from build123d import *

# Parameters (mm, degrees)
SKETCH_W     = 105
SKETCH_H     = 70
PAD_DEPTH    = 5
SKETCH001_R  = 6.375
POCKET_DEPTH = 5
SKETCH002_R  = 1.2
HOLE_DEPTH   = 25


with BuildPart() as part:
    # Sketch → Pad (new body)
    with BuildSketch(Plane.XY):
        Rectangle(SKETCH_W, SKETCH_H)
    extrude(amount=PAD_DEPTH)

    # Sketch001 (on Face6 of Pad) → Pocket (cut)
    with BuildSketch(Plane.XY.offset(5)):
        with Locations((-33, 11)):
            Circle(SKETCH001_R)
        with Locations((33, 11)):
            Circle(SKETCH001_R)
        with Locations((33, -11)):
            Circle(SKETCH001_R)
        with Locations((-33, -11)):
            Circle(SKETCH001_R)
        with Locations((-11, 11)):
            Circle(SKETCH001_R)
        with Locations((11, 11)):
            Circle(SKETCH001_R)
        with Locations((-11, -11)):
            Circle(SKETCH001_R)
        with Locations((11, -11)):
            Circle(SKETCH001_R)
    extrude(amount=-POCKET_DEPTH, mode=Mode.SUBTRACT)

    # Sketch002 (on Face5 of Pocket) → Hole (cut)
    with BuildSketch(Plane.XY.offset(5)):
        with Locations((-47.5, 32.5)):
            Circle(SKETCH002_R)
        with Locations((47.5, 32.5)):
            Circle(SKETCH002_R)
        with Locations((-47.5, -32.5)):
            Circle(SKETCH002_R)
        with Locations((47.5, -32.5)):
            Circle(SKETCH002_R)
    extrude(amount=-HOLE_DEPTH, mode=Mode.SUBTRACT)


solid = part.part
Here's how the part is built. I have some questions about the finished solid (model axes, mm). Round coordinates to 2 decimals unless told otherwise and drop trailing zeros. Order: outer loops, then holes, each group sorted by start corner. A loop starts at its lowest first (then second) coordinate and runs counter-clockwise, first axis right, second up. Notation, with made-up numbers: (-15.75, 81) -> (-7.75, 81) arc R23 ccw to (-7.75, 96) -> close; hole circle Ø10 at (50.5, 73). An arc over 180 degrees is marked (long way). Return JSON: item names as keys, results as strings.
Q1. For pin 1 Ø11.5 at (x, y) = (11, 11) entering from +Z, with a flat end and sliding along its axis, tell me the tip position at first contact or that it passes through.
Filled sheet:
{"pin 1": "passes through"}
Q2. If we section it at B-B on z = 2.5: Give the number of separate pieces and of enclosed holes in the cut face, plus the area to 3 significant figures.
Filled sheet:
{"separate pieces": "1", "enclosed holes": "12", "area": "6,310 mm^2"}
Q3. If we section it at C-C on x = -47.5: List the corners of the cut face in (y, z) for me.
Filled sheet:
{"outline": "(-35, 0) -> (-33.7, 0) -> (-33.7, 5) -> (-35, 5) -> close; (-31.3, 0) -> (31.3, 0) -> (31.3, 5) -> (-31.3, 5) -> close; (33.7, 0) -> (35, 0) -> (35, 5) -> (33.7, 5) -> close"}
Q4. If we section it at D-D on y = 11: List the corners of the cut face in (x, z) for me (3 decimals), plus the area to 3 significant figures.
Filled sheet:
{"outline": "(-52.5, 0) -> (-39.375, 0) -> (-39.375, 5) -> (-52.5, 5) -> close; (-26.625, 0) -> (-17.375, 0) -> (-17.375, 5) -> (-26.625, 5) -> close; (-4.625, 0) -> (4.625, 0) -> (4.625, 5) -> (-4.625, 5) -> close; (17.375, 0) -> (26.625, 0) -> (26.625, 5) -> (17.375, 5) -> close; (39.375, 0) -> (52.5, 0) -> (52.5, 5) -> (39.375, 5) -> close", "area": "270 mm^2"}
Q5. If we mould it in two halves opening along X, with no side actions, what happens to faces 1 (the flat face through (-1, 0, 5)), 2 (the cylindrical face through (-46.355, -32.14, 2.535)), 3 (the cylindrical face through (-46.355, 32.86, 2.535)), 4 (the flat face through (-52.5, 0, 2))? For each: released by +X, released by -X, zero draft, split by the parting line, or undercut.
Filled sheet:
{"face 1": "zero draft", "face 2": "undercut", "face 3": "undercut", "face 4": "released by -X"}
Q6. If we section it at A-A on y = 32.5: List the corners of the cut face in (x, z) for me, plus the area to 3 significant figures.
Filled sheet:
{"outline": "(-52.5, 0) -> (-48.7, 0) -> (-48.7, 5) -> (-52.5, 5) -> close; (-46.3, 0) -> (46.3, 0) -> (46.3, 5) -> (-46.3, 5) -> close; (48.7, 0) -> (52.5, 0) -> (52.5, 5) -> (48.7, 5) -> close", "area": "501 mm^2"}
Q7. I need wall thicknesses on line 1 along X through (y, z) = (-10.5, 4.45); line 2 along Y through (x, z) = (33, 3.25) (3 decimals); line 3 along Y through (x, z) = (36, 2.85) (3 decimals). Which ranges of each line are inside material? Lowest first, please. Write a range as from..to.
Filled sheet:
{"line 1": "x = -52.5..-39.36, -26.64..-17.36, -4.64..4.64, 17.36..26.64, 39.36..52.5", "line 2": "y = -35..-17.375, -4.625..4.625, 17.375..35", "line 3": "y = -35..-16.625, -5.375..5.375, 16.625..35"}
